Read the model definition and answer for the solid it produces. Units are mm, in the model's axes. Face numbers are marked on the shaded views. A direction names the side the tool comes from. Give positions to 0.01 mm unless a question says otherwise; leave off trailing zeros. Order: outer loops, then holes, each group sorted by start corner. A loop starts at its lowest first (then second) coordinate and runs counter-clockwise, first axis right, second up. Notation, with made-up numbers: M 29.25,0 L 72.25,0 A19 ccw 72.25,16 Z; hole C 60,-2 d5. An arc over 180 degrees is marked long. One line per item, written item: value. Start each with the question number.
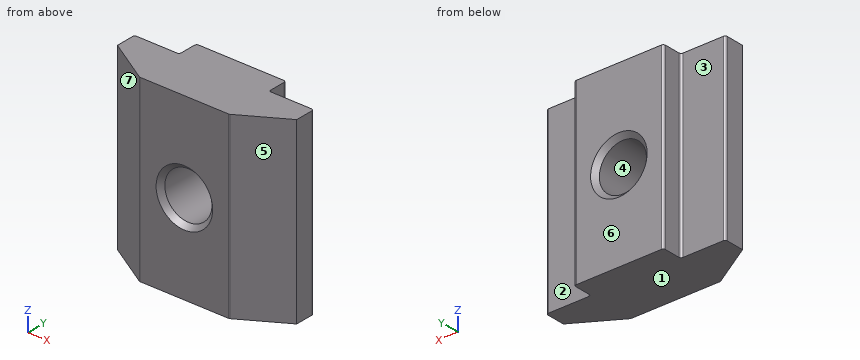
from build123d import *

# Parameters (mm, degrees)
EXTRUDE_1_DEPTH = 8
FILLET_1_R      = 0.2


with BuildPart() as part:
    # Эскиз1 → Бобышка-Вытянуть1 (new body, symmetric)
    with BuildSketch(Plane.XY):
        Polygon((4, 0), (-4, 0), (-4, -1.8), (-8, -1.8), (-8, -3.6), (-4, -6), (4, -6), (8, -3.6), (8, -1.8), (4, -1.8), align=None)
    extrude(amount=EXTRUDE_1_DEPTH, both=True)

    # Эскиз4 → Отверстие обработанное метчиком M52 (revolve, cut)
    with BuildSketch(Plane(origin=(0, 0, 0), x_dir=(0, 0, 1), z_dir=(1, 0, 0))):
        Polygon((0, 0), (0, 6), (2.525, 6), (2.1, 5.575), (2.1, 0.425), (2.525, 0), align=None)
    revolve(axis=Axis((0, 6.35, 0), (0, -1, 0)), mode=Mode.SUBTRACT)

    # Скругление1
    fillet_1_edges = [part.edges().sort_by_distance(p)[0] for p in [
        (-4, 0, 0),
        (4, 0, 0),
        (4, -1.8, 0),
        (8, -1.8, 0),
        (4, -6, 0),
        (-4, -6, 0),
        (-8, -1.8, 0),
        (-4, -1.8, 0),
    ]]
    fillet(fillet_1_edges, radius=FILLET_1_R)


solid = part.part
Q1. A tool of negligible diameter and unlimited length cuts with its end or side. For the marked faces 1, 2 and 3, from which of +Z, -Z, +X, -X, +Y, -Y can it reach the whole face along a straight path? Write none if from no direction.
Q2. Consider probe 1 along Z at (x, y) = (0, -2.5); probe 2 along X at (y, z) = (-0.85, -5.75). Determine where each line is inside the solid, lowest interval first.
Q3. Each of these flat-tipped pins is pushed along its axis until it touches: pin 1 (3 mm diameter, centred on x = -6.5, z = -0.5, fed in from +Y); pin 2 (2.5 mm diameter, centred on x = 0, z = 0, fed in from +Y); pin 3 (0.7 mm diameter, centred on y = -1, z = -1, fed in from -X); pin 4 (3 mm diameter, centred on x = -1, z = 0, fed in from -Y) (3 decimals). Where does it stop, or does it pass through?
Q4. Find section A-A, the plane x = 0. Give the vertices of the cut face in (y, z) (3 decimals).
Q5. Find section C-C, the plane z = 4.25. Give the vertices of the cut face in (x, y), then the cut area to 3 significant figures.
Q6. Determine the mould class of the marked faces 4, 5, 6 and 7 for opening direction X: released by +X, released by -X, zero draft, split by the parting line, or undercut.
Q7. Find section D-D, the plane y = -0.65. Give the vertices of the cut face in (x, z), then the cut area to 3 significant figures.
Evaluation:
1. face 1: -Z, +X, -X, +Y, -Y
1. face 2: +Z, -Z, +X, +Y
1. face 3: +Z, -Z, -X, +Y
2. probe 1: -8 to -2.1, 2.1 to 8
2. probe 2: -4 to 4
3. pin 1: y = -1.8
3. pin 2: through
3. pin 3: x = -4
3. pin 4: y = -5.975
4. outline: M -6,-8 L 0,-8 L 0,-2.525 L -0.425,-2.1 L -5.575,-2.1 L -6,-2.525 Z; M -6,2.525 L -5.575,2.1 L -0.425,2.1 L 0,2.525 L 0,8 L -6,8 Z
5. outline: M -8,-3.6 L -4.05,-5.97 A0.2 ccw -3.94,-6 L 3.94,-6 A0.2 ccw 4.05,-5.97 L 8,-3.6 L 8,-2 A0.2 ccw 7.8,-1.8 L 4.2,-1.8 A0.2 cw 4,-1.6 L 4,-0.2 A0.2 ccw 3.8,0 L -3.8,0 A0.2 ccw -4,-0.2 L -4,-1.6 A0.2 cw -4.2,-1.8 L -7.8,-1.8 A0.2 ccw -8,-2 Z
5. area: 72.0 mm2
6. face 4: undercut
6. face 5: released by +X
6. face 6: zero draft
6. face 7: released by -X
7. outline: M -4,-8 L 4,-8 L 4,8 L -4,8 Z; hole C 0,0 d4.2
7. area: 114 mm2
